```python
from build123d import *

# Parameters (mm, degrees)
SKETCH1_W            = 300
SKETCH1_H            = 213
BOSS_EXTRUDE1_DEPTH  = 3
SKETCH2_W            = 3
SKETCH2_H            = 21
CUT_EXTRUDE1_DEPTH   = 184.987091939
SKETCH3_W            = 20
SKETCH3_H            = 3
SKETCH3_W_2          = 10
CUT_EXTRUDE2_DEPTH   = 184.987091939
SKETCH4_W            = 3
SKETCH4_H            = 20
CUT_EXTRUDE3_DEPTH   = 184.987091939
SKETCH6_R            = 1.3
CUT_EXTRUDE4_DEPTH   = 184.987091939
CUT_EXTRUDE5_DEPTH   = 184.987091939
FILLET1_R            = 4
FILLET1_OF_MIRROR1_R = 4
SKETCH8_R            = 1.3
CUT_EXTRUDE6_DEPTH   = 184.987091939
CUT_EXTRUDE7_DEPTH   = 184.987091939
CUT_EXTRUDE8_DEPTH   = 157.208994619
FILLET2_R            = 2
SKETCH11_W           = 183
SKETCH11_H           = 8
CUT_EXTRUDE9_DEPTH   = 157.208994619
FILLET3_R            = 22


with BuildPart() as part:
    # Sketch1 → Boss-Extrude1 (new body)
    with BuildSketch(Plane(origin=(0, 0, 0), x_dir=(1, 0, 0), z_dir=(0, 1, 0))):
        Rectangle(SKETCH1_W, SKETCH1_H)
    extrude(amount=BOSS_EXTRUDE1_DEPTH)

    # Sketch2 → Cut-Extrude1 (cut, through all)
    with BuildSketch(Plane(origin=(0, 3, 0), x_dir=(1, 0, 0), z_dir=(0, 1, 0))):
        with Locations((-148.5, 96)):
            Rectangle(SKETCH2_W, SKETCH2_H)
        Polygon((-150, -13.5), (-150, 0), (-150, 13.5), (-147, 13.5), (-147, -13.5), align=None)
        with Locations((-148.5, 54)):
            Rectangle(SKETCH2_W, SKETCH2_H)
        with Locations((-148.5, -54)):
            Rectangle(SKETCH2_W, SKETCH2_H)
        with Locations((-148.5, -96)):
            Rectangle(SKETCH2_W, SKETCH2_H)
    extrude(amount=-CUT_EXTRUDE1_DEPTH, mode=Mode.SUBTRACT)

    # Sketch3 → Cut-Extrude2 (cut, through all)
    with BuildSketch(Plane(origin=(0, 3, 0), x_dir=(1, 0, 0), z_dir=(0, 1, 0))):
        with Locations((-137, 21.5)):
            Rectangle(SKETCH3_W, SKETCH3_H)
        with Locations((-64, 21.5)):
            Rectangle(SKETCH3_W_2, SKETCH3_H)
        with Locations((9, 21.5)):
            Rectangle(SKETCH3_W, SKETCH3_H)
        with Locations((9, -21.5)):
            Rectangle(SKETCH3_W, SKETCH3_H)
        with Locations((-64, -21.5)):
            Rectangle(SKETCH3_W_2, SKETCH3_H)
        with Locations((-137, -21.5)):
            Rectangle(SKETCH3_W, SKETCH3_H)
    extrude(amount=-CUT_EXTRUDE2_DEPTH, mode=Mode.SUBTRACT)

    # Sketch4 → Cut-Extrude3 (cut, through all)
    with BuildSketch(Plane(origin=(0, 3, 0), x_dir=(1, 0, 0), z_dir=(0, 1, 0))):
        with Locations((20.5, 0)):
            Rectangle(SKETCH4_W, SKETCH4_H)
    extrude(amount=-CUT_EXTRUDE3_DEPTH, mode=Mode.SUBTRACT)

    # Sketch6 → Cut-Extrude4 (cut, through all)
    with BuildSketch(Plane(origin=(0, 3, 0), x_dir=(1, 0, 0), z_dir=(0, 1, 0))):
        with Locations(Location((-137, 32, 0), (0, 0, 270))):
            Circle(SKETCH6_R)
        with Locations(Location((-64, 32, 0), (0, 0, 270))):
            Circle(SKETCH6_R)
        with Locations(Location((9, 32, 0), (0, 0, 270))):
            Circle(SKETCH6_R)
        with Locations(Location((9, -32, 0), (0, 0, 270))):
            Circle(SKETCH6_R)
        with Locations(Location((-64, -32, 0), (0, 0, 270))):
            Circle(SKETCH6_R)
        with Locations(Location((-137, -32, 0), (0, 0, 270))):
            Circle(SKETCH6_R)
    extrude(amount=-CUT_EXTRUDE4_DEPTH, mode=Mode.SUBTRACT)

    # Sketch7 → Cut-Extrude5 (cut, through all)
    with BuildSketch(Plane(origin=(0, 3, 0), x_dir=(1, 0, 0), z_dir=(0, 1, 0))):
        Polygon((-115, 90), (-115, 60), (-85, 60), align=None)
        Polygon((-108, 90), (-78, 60), (-78, 90), align=None)
        Polygon((-64, 90), (-34, 90), (-64, 60), align=None)
        Polygon((-27, 60), (-57, 60), (-27, 90), align=None)
        Polygon((-15, 90), (-15, 60), (15, 60), align=None)
        Polygon((-8, 90), (22, 60), (22, 90), align=None)
        Polygon((36, 90), (66, 90), (36, 60), align=None)
        Polygon((73, 60), (43, 60), (73, 90), align=None)
        Polygon((85, 90), (85, 60), (115, 60), align=None)
        Polygon((92, 90), (122, 60), (122, 90), align=None)
    cut_extrude5 = extrude(amount=-CUT_EXTRUDE5_DEPTH, mode=Mode.SUBTRACT)

    # Fillet1
    fillet1_edges = [part.edges().sort_by_distance(p)[0] for p in [
        (-115, 1.5, -90),
        (-85, 1.5, -60),
        (-115, 1.5, -60),
        (-8, 1.5, -90),
        (22, 1.5, -90),
        (22, 1.5, -60),
        (36, 1.5, -60),
        (36, 1.5, -90),
        (66, 1.5, -90),
        (73, 1.5, -90),
        (73, 1.5, -60),
        (43, 1.5, -60),
        (92, 1.5, -90),
        (122, 1.5, -90),
        (122, 1.5, -60),
        (85, 1.5, -90),
        (115, 1.5, -60),
        (85, 1.5, -60),
        (-108, 1.5, -90),
        (-78, 1.5, -90),
        (-78, 1.5, -60),
        (-64, 1.5, -60),
        (-64, 1.5, -90),
        (-34, 1.5, -90),
        (-27, 1.5, -90),
        (-27, 1.5, -60),
        (-57, 1.5, -60),
        (-15, 1.5, -90),
        (15, 1.5, -60),
        (-15, 1.5, -60),
    ]]
    fillet(fillet1_edges, radius=FILLET1_R)

    # Mirror1: Cut-Extrude5 across plane
    add(cut_extrude5.mirror(Plane.XY), mode=Mode.SUBTRACT)

    # Fillet1 of Mirror1
    fillet1_of_mirror1_edges = [part.edges().sort_by_distance(p)[0] for p in [
        (-115, 1.5, 90),
        (-85, 1.5, 60),
        (-115, 1.5, 60),
        (-8, 1.5, 90),
        (22, 1.5, 90),
        (22, 1.5, 60),
        (36, 1.5, 60),
        (36, 1.5, 90),
        (66, 1.5, 90),
        (73, 1.5, 90),
        (73, 1.5, 60),
        (43, 1.5, 60),
        (92, 1.5, 90),
        (122, 1.5, 90),
        (122, 1.5, 60),
        (85, 1.5, 90),
        (115, 1.5, 60),
        (85, 1.5, 60),
        (-108, 1.5, 90),
        (-78, 1.5, 90),
        (-78, 1.5, 60),
        (-64, 1.5, 60),
        (-64, 1.5, 90),
        (-34, 1.5, 90),
        (-27, 1.5, 90),
        (-27, 1.5, 60),
        (-57, 1.5, 60),
        (-15, 1.5, 90),
        (15, 1.5, 60),
        (-15, 1.5, 60),
    ]]
    fillet(fillet1_of_mirror1_edges, radius=FILLET1_OF_MIRROR1_R)

    # Sketch8 → Cut-Extrude6 (cut, through all)
    with BuildSketch(Plane(origin=(0, 3, 0), x_dir=(1, 0, 0), z_dir=(0, 1, 0))):
        with Locations(Location((-136.98744233, -10, 0), (0, 0, 270))):
            Circle(SKETCH8_R)
        with Locations(Location((-64, -10, 0), (0, 0, 270))):
            Circle(SKETCH8_R)
        with Locations(Location((9, -10, 0), (0, 0, 270))):
            Circle(SKETCH8_R)
        with Locations(Location((-136.98744233, 10, 0), (0, 0, 90))):
            Circle(SKETCH8_R)
        with Locations(Location((-64, 10, 0), (0, 0, 90))):
            Circle(SKETCH8_R)
        with Locations(Location((9, 10, 0), (0, 0, 90))):
            Circle(SKETCH8_R)
    extrude(amount=-CUT_EXTRUDE6_DEPTH, mode=Mode.SUBTRACT)

    # Sketch9 → Cut-Extrude7 (cut, through all)
    with BuildSketch(Plane(origin=(0, 3, 0), x_dir=(1, 0, 0), z_dir=(0, 1, 0))):
        Polygon((-147, 43.5), (33, 43.5), (33, -43.5), (-147, -43.5), (-187.25008624, -43.5), (-187.25008624, -148.565138747), (177.736932827, -148.565138747), (177.736932827, 142.910410283), (-187.25008624, 142.910410283), (-187.25008624, 43.5), align=None)
    extrude(amount=-CUT_EXTRUDE7_DEPTH, mode=Mode.SUBTRACT)

    # Sketch10 → Cut-Extrude8 (cut, through all)
    with BuildSketch(Plane(origin=(0, 3, 0), x_dir=(1, 0, 0), z_dir=(0, 1, 0))):
        Polygon((-123, 16), (-98, 16), (-98, -14), align=None)
        Polygon((-92, 16), (-92, -14), (-67, 16), align=None)
        Polygon((-124.333333333, 4), (-124.333333333, -14), (-109.333333333, -14), align=None)
        Polygon((-80.666666667, -14), (-65.666666667, 4), (-65.666666667, -14), align=None)
        Polygon((-62.333333333, 4), (-62.333333333, -14), (-47.333333333, -14), align=None)
        Polygon((-18.666666667, -14), (-3.666666667, 4), (-3.666666667, -14), align=None)
        Polygon((-61, 16), (-36, 16), (-36, -14), align=None)
        Polygon((-30, -14), (-5, 16), (-30, 16), align=None)
    extrude(amount=-CUT_EXTRUDE8_DEPTH, mode=Mode.SUBTRACT)

    # Fillet2
    fillet2_edges = [part.edges().sort_by_distance(p)[0] for p in [
        (-98, 1.5, 14),
        (-123, 1.5, -16),
        (-98, 1.5, -16),
        (-65.666666667, 1.5, 14),
        (-80.666666667, 1.5, 14),
        (-65.666666667, 1.5, -4),
        (-124.333333333, 1.5, -4),
        (-109.333333333, 1.5, 14),
        (-124.333333333, 1.5, 14),
        (-92, 1.5, -16),
        (-67, 1.5, -16),
        (-92, 1.5, 14),
        (-30, 1.5, 14),
        (-30, 1.5, -16),
        (-5, 1.5, -16),
        (-36, 1.5, 14),
        (-61, 1.5, -16),
        (-36, 1.5, -16),
        (-3.666666667, 1.5, 14),
        (-18.666666667, 1.5, 14),
        (-3.666666667, 1.5, -4),
        (-62.333333333, 1.5, -4),
        (-47.333333333, 1.5, 14),
        (-62.333333333, 1.5, 14),
    ]]
    fillet(fillet2_edges, radius=FILLET2_R)

    # Sketch11 → Cut-Extrude9 (cut, through all)
    with BuildSketch(Plane(origin=(0, 3, 0), x_dir=(1, 0, 0), z_dir=(0, 1, 0))):
        with Locations((-58.5, 39.5)):
            Rectangle(SKETCH11_W, SKETCH11_H)
        with Locations((-58.5, -39.5)):
            Rectangle(SKETCH11_W, SKETCH11_H)
    extrude(amount=-CUT_EXTRUDE9_DEPTH, mode=Mode.SUBTRACT)

    # Fillet3
    fillet3_edges = [part.edges().sort_by_distance(p)[0] for p in [
        (33, 1.5, -35.5),
        (33, 1.5, 35.5),
    ]]
    fillet(fillet3_edges, radius=FILLET3_R)


solid = part.part
```
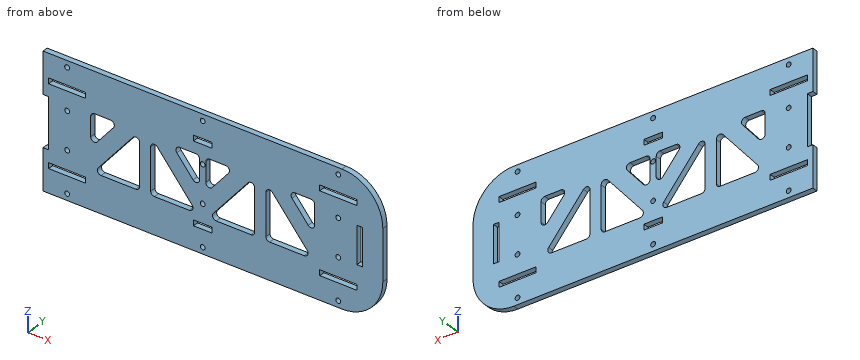
Could you check a few things on this model? Use its own coordinates, in mm. Coordinates: 2 decimals unless noted, no trailing zeros. Order: outer loops, then holes, each group sorted by start corner. A loop starts at its lowest first (then second) coordinate and runs counter-clockwise, first axis right, second up. Notation, with made-up numbers: M 56.5,-25 L 95.5,-25 A22 ccw 95.5,-10 Z; hole C 72,-4.5 d1. An arc over 180 degrees is marked long. Use a Markdown table: item, result. Add a question column.
Q1. If I drill on L1, parallel to Z at x = 2, y = 0.5; L2, parallel to X at y = 2.7, z = -6.5; L3, parallel to X at y = 2.05, z = -2, over which ranges is the centre line in solid material (lowest first)?
Q2. I want a section at D-D on z = -29. List the corners of the cut face in (x, y) for me, then the cut area to 3 significant figures.
Q3. I'm going to push flat-ended pins straight in: pin 1 (2.5 mm diameter, centred on x = -64, z = 32, fed in from -Y); pin 2 (1.5 mm diameter, centred on y = 1.5, z = 22, fed in from +X). Where does each tip first touch, or does it pass through?
Q4. I want a section at C-C on y = 2.3. Give the number of separate pieces and of enclosed holes in the cut face, then the cut area to 3 significant figures.
Q5. I want a section at A-A on x = 3. List the corners of the cut face in (y, z) for me, then the cut area to 3 significant figures.
Q6. I want a section at B-B on z = -3. List the corners of the cut face in (x, y) for me.
Checked values:
| question | item | result |
|---|---|---|
| 1 | L1 | -35.5 to -23, -20 to 20, 23 to 35.5 |
| 1 | L2 | -147 to -115.08, -98 to -92, -74.92 to -53.08, -36 to -30, -12.92 to 19, 22 to 33 |
| 1 | L3 | -147 to -111.33, -98 to -92, -78.67 to -49.33, -36 to -30, -16.67 to 19, 22 to 33 |
| 2 | outline | M -150,0 L 26.61,0 L 26.61,3 L -150,3 Z |
| 2 | area | 530 mm² |
| 3 | pin 1 | through |
| 3 | pin 2 | x = 31.59 |
| 4 | separate pieces | 1 |
| 4 | enclosed holes | 27 |
| 4 | area | 10,300 mm² |
| 5 | outline | M 0,-35.5 L 3,-35.5 L 3,-23 L 0,-23 Z; M 0,-20 L 3,-20 L 3,20 L 0,20 Z; M 0,23 L 3,23 L 3,35.5 L 0,35.5 Z |
| 5 | area | 195 mm² |
| 6 | outline | M -147,0 L -112.17,0 L -112.17,3 L -147,3 Z; M -98,0 L -92,0 L -92,3 L -98,3 Z; M -77.83,0 L -50.17,0 L -50.17,3 L -77.83,3 Z; M -36,0 L -30,0 L -30,3 L -36,3 Z; M -15.83,0 L 19,0 L 19,3 L -15.83,3 Z; M 22,0 L 33,0 L 33,3 L 22,3 Z |
